Source: CAD feature listing. Evaluate the final solid. Frame: model axes, mm. A direction names the side the tool comes from. Give positions to 0.01 mm unless a question says otherwise; leave off trailing zeros. Write each loop counter-clockwise with the first axis right and the second up, starting at its lowest first coordinate (ties: lowest second). Pieces come first, ordered by that corner, then holes. Notation, with made-up numbers: M -33.5,-27 L -8.5,-27 A28 ccw -8.5,12 Z; hole C 69.5,87.25 d7. An arc over 180 degrees is marked long. Return JSON: item names as keys, results as strings.
```python
from build123d import *

# Parameters (mm, degrees)
SKETCH016_W     = 238
SKETCH016_H     = 288
PAD006_DEPTH    = 18
SKETCH018_W     = 6
SKETCH018_H     = 12
POCKET010_DEPTH = 238
SKETCH017_W     = 6
SKETCH017_H     = 12
POCKET011_DEPTH = 288
SKETCH019_R     = 6
POCKET012_DEPTH = 18
SKETCH020_R     = 12.75
POCKET013_DEPTH = 2.4


with BuildPart() as part:
    # Sketch016 → Pad006 (new body)
    with BuildSketch(Plane.XY):
        with Locations((0, 144)):
            Rectangle(SKETCH016_W, SKETCH016_H)
    extrude(amount=PAD006_DEPTH)

    # Sketch018 → Pocket010 (cut)
    with BuildSketch(Plane(origin=(-119, 0, 0), x_dir=(0, -1, 0), z_dir=(-1, 0, 0))):
        with Locations((-285, 6)):
            Rectangle(SKETCH018_W, SKETCH018_H)
    extrude(amount=-POCKET010_DEPTH, mode=Mode.SUBTRACT)

    # Sketch017 → Pocket011 (cut)
    with BuildSketch(Plane.XZ):
        with Locations((-116, 6)):
            Rectangle(SKETCH017_W, SKETCH017_H)
    pocket011 = extrude(amount=-POCKET011_DEPTH, mode=Mode.SUBTRACT)

    # Mirrored001: Pocket011 across Sketch017 V_Axis
    add(pocket011.mirror(Plane(origin=(0, 0, 0), x_dir=(0, -1, 0), z_dir=(1, 0, 0))), mode=Mode.SUBTRACT)

    # Sketch019 → Pocket012 (cut)
    with BuildSketch(Plane.XY.offset(18)):
        with Locations((-85, 63)):
            Circle(SKETCH019_R)
        with Locations((-85, 233)):
            Circle(SKETCH019_R)
        with Locations((85, 233)):
            Circle(SKETCH019_R)
        with Locations((85, 63)):
            Circle(SKETCH019_R)
    extrude(amount=-POCKET012_DEPTH, mode=Mode.SUBTRACT)

    # Sketch020 → Pocket013 (cut)
    with BuildSketch(Plane.XY.offset(18)):
        with Locations((-85, 63)):
            Circle(SKETCH020_R)
        with Locations((85, 63)):
            Circle(SKETCH020_R)
        with Locations((85, 233)):
            Circle(SKETCH020_R)
        with Locations((-85, 233)):
            Circle(SKETCH020_R)
    extrude(amount=-POCKET013_DEPTH, mode=Mode.SUBTRACT)


solid = part.part
```
1) Cut plane B-B, the plane z = 9. Return the cut outline in (x, y), then the cut area to 3 significant figures.
Numbers:
{"outline": "M -113,0 L 113,0 L 113,282 L -113,282 Z; hole C -85,63 d12; hole C -85,233 d12; hole C 85,63 d12; hole C 85,233 d12", "area": "63,300 mm²"}
2) Cut plane C-C, the plane y = 233. Return the cut outline in (x, z), then the cut area to 3 significant figures.
Numbers:
{"outline": "M -119,12 L -113,12 L -113,0 L -91,0 L -91,15.6 L -97.75,15.6 L -97.75,18 L -119,18 Z; M -79,0 L 79,0 L 79,15.6 L 72.25,15.6 L 72.25,18 L -72.25,18 L -72.25,15.6 L -79,15.6 Z; M 91,0 L 113,0 L 113,12 L 119,12 L 119,18 L 97.75,18 L 97.75,15.6 L 91,15.6 Z", "area": "3,640 mm²"}
3) Contact query for flat-ended pins moving along their axis: pin 1 Ø1.5 at (x, z) = (-70.5, 9.5) entering from -Y; pin 2 Ø1.5 at (y, z) = (258.5, 4) entering from +X; pin 3 Ø3.5 at (x, z) = (-48.5, 6.5) entering from +Y; pin 4 Ø20.5 at (x, y) = (-85, 233) entering from +Z. Output: stop coordinate, or through.
Numbers:
{"pin 1": "stops at y = 0", "pin 2": "stops at x = 113", "pin 3": "stops at y = 282", "pin 4": "stops at z = 15.6"}
4) Draft query along X for faces 1 (the face through (-85.78, 238.95, 7.91)), 2 (the face through (-2, 146, 18)), 3 (the face through (119, 142, 15)). Return one class per face: released by +X, released by -X, zero draft, split by the parting line, or undercut.
Numbers:
{"face 1": "undercut", "face 2": "zero draft", "face 3": "released by +X"}
5) Set-up query: faces 4 (the face through (-2, 282, 6)), 5 (the face through (-88, 57.5, 15.6)), 6 (the face through (-119, 142, 15)), 7 (the face through (113, 139, 6)), 8 (the face through (-113, 139, 6)). Return all of +Z, -Z, +X, -X, +Y, -Y with unobstructed straight access to the full face (end or side cutting, diameter ignored); none if empty.
Numbers:
{"face 4": "-Z, +X, -X, +Y", "face 5": "+Z", "face 6": "+Z, -Z, -X, +Y, -Y", "face 7": "-Z, +X, +Y, -Y", "face 8": "-Z, -X, +Y, -Y"}
6) Cut plane D-D, the plane y = 85. Return the cut outline in (x, z), then the cut area to 3 significant figures.
Numbers:
{"outline": "M -119,12 L -113,12 L -113,0 L 113,0 L 113,12 L 119,12 L 119,18 L -119,18 Z", "area": "4,140 mm²"}
7) Line query: line 1 (Y direction, x = 85, z = 9.75); line 2 (Y direction, x = -85, z = 17.5); line 3 (X direction, y = 62.5, z = 16.75). Output: solid intervals per line, ascending. Write a range as [from, to].
Numbers:
{"line 1": "y = [0, 57], [69, 227], [239, 282]", "line 2": "y = [0, 50.25], [75.75, 220.25], [245.75, 288]", "line 3": "x = [-119, -97.74], [-72.26, 72.26], [97.74, 119]"}
8) Cut plane A-A, the plane x = 85. Return the cut outline in (y, z), then the cut area to 3 significant figures.
Numbers:
{"outline": "M 0,0 L 57,0 L 57,15.6 L 50.25,15.6 L 50.25,18 L 0,18 Z; M 69,0 L 227,0 L 227,15.6 L 220.25,15.6 L 220.25,18 L 75.75,18 L 75.75,15.6 L 69,15.6 Z; M 239,0 L 282,0 L 282,12 L 288,12 L 288,18 L 245.75,18 L 245.75,15.6 L 239,15.6 Z", "area": "4,620 mm²"}
